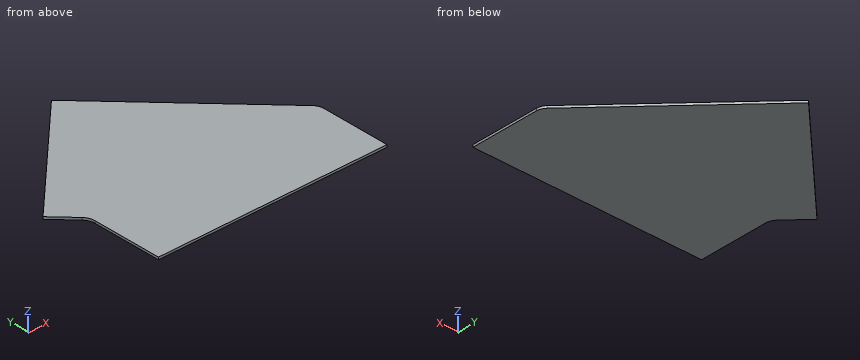
```python
from build123d import *

# Parameters (mm, degrees)
EXTRUDE_2_DEPTH = 2
FILLET_1_R      = 10
FILLET_2_R      = 12


with BuildPart() as part:
    # Эскиз2 → Бобышка-Вытянуть2 (new body)
    with BuildSketch(Plane.XY):
        Polygon((0, 0), (200, 0), (200, 64), (78.286796564, 185.713203436), (-21.213203436, 86.213203436), (0, 65), align=None)
    extrude(amount=EXTRUDE_2_DEPTH)

    # Скругление1
    fillet_1_edges = [part.edges().sort_by_distance(p)[0] for p in [
        (200, 64, 1),
    ]]
    fillet(fillet_1_edges, radius=FILLET_1_R)

    # Скругление2
    fillet_2_edges = [part.edges().sort_by_distance(p)[0] for p in [
        (0, 65, 1),
    ]]
    fillet(fillet_2_edges, radius=FILLET_2_R)


solid = part.part
```
Here's how the part is built. I have some questions about the finished solid (model axes, mm). Round coordinates to 2 decimals unless told otherwise and drop trailing zeros. Order: outer loops, then holes, each group sorted by start corner. A loop starts at its lowest first (then second) coordinate and runs counter-clockwise, first axis right, second up. Notation, with made-up numbers: (64.25, -16.5) -> (112.25, -16.5) arc R9 ccw to (112.25, -1.5) -> close; hole circle Ø9 at (55, 30.5). An arc over 180 degrees is marked (long way). Use a Markdown table: item, result. Add a question column.
(1) I need wall thicknesses on line 1 along X through (y, z) = (55, 1.05); line 2 along X through (y, z) = (132.5, 1.45); line 3 along Y through (x, z) = (3, 0.4). Which ranges of each line are inside material? Lowest first, please.
(2) For pin 1 Ø0.6 at (y, z) = (17.5, 1) entering from -X; pin 2 Ø1 at (y, z) = (99, 1.5) entering from -X, each with a flat end and sliding along its axis, tell me the tip position at first contact or that it passes through.
(3) Suppose I cut it at B-B, the plane x = 118.5. Please give me the cut outline in (y, z).
(4) Suppose I cut it at A-A, the plane z = 1.45. Please give me the cut outline in (x, y), and give its area (3 significant figures).
(5) Suppose I cut it at C-C, the plane y = 40.5. Please give me the cut outline in (x, z).
Verdict:
| question | item | result |
|---|---|---|
| 1 | line 1 | 0 to 200 |
| 1 | line 2 | 25.07 to 131.5 |
| 1 | line 3 | 0 to 110.43 |
| 2 | pin 1 | x = 0 |
| 2 | pin 2 | x = -8.93 |
| 3 | outline | (0, 0) -> (145.5, 0) -> (145.5, 2) -> (0, 2) -> close |
| 4 | outline | (-21.21, 86.21) -> (-3.51, 68.51) arc R12 cw to (0, 60.03) -> (0, 0) -> (200, 0) -> (200, 59.86) arc R10 ccw to (197.07, 66.93) -> (78.29, 185.71) -> close |
| 4 | area | 27,100 mm2 |
| 5 | outline | (0, 0) -> (200, 0) -> (200, 2) -> (0, 2) -> close |
